Part model, mm, in its own coordinate system. Face numbers are marked on the shaded views. A direction names the side the tool comes from. Round coordinates to 2 decimals unless told otherwise and drop trailing zeros. Order: outer loops, then holes, each group sorted by start corner. A loop starts at its lowest first (then second) coordinate and runs counter-clockwise, first axis right, second up. Notation, with made-up numbers: (40.5, 67.5) -> (48.5, 67.5) arc R23 ccw to (48.5, 75.5) -> close; hole circle Ø9 at (88, -15.5). An arc over 180 degrees is marked (long way). Use CSV: the item, a comma, the result in double quotes.
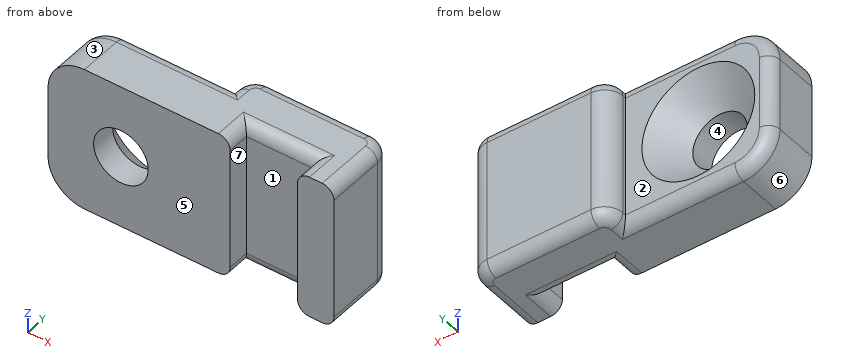
```python
from build123d import *

# Parameters (mm, degrees)
RESSALTO_EXTRUS_O1_DEPTH = 8
ESBO_O2_R                = 1.5
CORTE_EXTRUS_O1_DEPTH    = 6
CHANFRO2_SIZE            = 1.6
FILETE3_R                = 2
FILETE5_R                = 1
FILETE6_R                = 0.65


with BuildPart() as part:
    # Esboço1 → Ressalto-extrusão1 (new body)
    with BuildSketch(Plane.XY):
        Polygon((-11.5, -1.2), (-11.5, 1.8), (-3.5, 1.8), (-3.5, 3), (4.2, 3), (4.2, -1.2), (2.2, -1.2), (2.2, 0), (-1.5, 0), (-1.5, -1.2), align=None)
    extrude(amount=RESSALTO_EXTRUS_O1_DEPTH)

    # Esboço2 → Corte-extrusão1 (cut)
    with BuildSketch(Plane(origin=(0, 1.8, 0), x_dir=(1, 0, 0), z_dir=(0, 1, 0))):
        with Locations(Location((-7.5, -4, 0), (0, 0, 180))):
            Circle(ESBO_O2_R)
    extrude(amount=-CORTE_EXTRUS_O1_DEPTH, mode=Mode.SUBTRACT)

    # Chanfro2
    chanfro2_edges = [part.edges().sort_by_distance(p)[0] for p in [
        (-6, 1.8, 4),
    ]]
    chamfer(chanfro2_edges, length=CHANFRO2_SIZE)

    # Filete3
    filete3_edges = [part.edges().sort_by_distance(p)[0] for p in [
        (-11.5, 0.3, 0),
        (-11.5, 0.3, 8),
    ]]
    fillet(filete3_edges, radius=FILETE3_R)

    # Filete5
    filete5_edges = [part.edges().sort_by_distance(p)[0] for p in [
        (-3.5, 3, 4),
        (4.2, 3, 4),
    ]]
    fillet(filete5_edges, radius=FILETE5_R)

    # Filete6
    filete6_edges = [part.edges().sort_by_distance(p)[0] for p in [
        (-1.5, -0.6, 0),
        (-6.5, 1.8, 0),
        (4.2, 0.4, 0),
        (2.2, -0.6, 0),
        (0.35, 0, 0),
        (4.2, 0.4, 8),
        (-6.5, 1.8, 8),
        (-1.5, -0.6, 8),
        (-11.5, 1.8, 4),
        (-10.914213562, 1.8, 0.585786438),
        (-10.914213562, 1.8, 7.414213562),
        (0.35, 0, 8),
        (-3.5, 1.9, 0),
        (-3.5, 1.9, 8),
        (0.35, 3, 0),
        (3.907106781, 2.707106781, 0),
        (-3.207106781, 2.707106781, 0),
        (0.35, 3, 8),
        (3.907106781, 2.707106781, 8),
        (-3.207106781, 2.707106781, 8),
        (2.2, -0.6, 8),
    ]]
    fillet(filete6_edges, radius=FILETE6_R)


solid = part.part
```
(1) Cut at A-A, the plane y = -0.2. Give the cut face in (x, z).
Reply:
outline,"(-11.5, 2) arc R2 ccw to (-9.5, 0) -> (-2.15, 0) arc R0.65 ccw to (-1.5, 0.65) -> (-1.5, 7.35) arc R0.65 ccw to (-2.15, 8) -> (-9.5, 8) arc R2 ccw to (-11.5, 6) -> close; (2.2, 0.65) arc R0.65 ccw to (2.85, 0) -> (3.55, 0) arc R0.65 ccw to (4.2, 0.65) -> (4.2, 7.35) arc R0.65 ccw to (3.55, 8) -> (2.85, 8) arc R0.65 ccw to (2.2, 7.35) -> close; hole circle Ø3 at (-7.5, 4)"
(2) Cut at D-D, the plane x = 1.5. Give the cut face in (y, z).
Reply:
outline,"(0, 0.65) arc R0.65 ccw to (0.65, 0) -> (2.35, 0) arc R0.65 ccw to (3, 0.65) -> (3, 7.35) arc R0.65 ccw to (2.35, 8) -> (0.65, 8) arc R0.65 ccw to (0, 7.35) -> close"
(3) Cut at C-C, the plane z = 4. Give the cut face in (x, y).
Reply:
outline,"(-11.5, -1.2) -> (-9, -1.2) -> (-9, 0.2) -> (-10.6, 1.8) -> (-10.85, 1.8) arc R0.65 ccw to (-11.5, 1.15) -> close; (-6, -1.2) -> (-1.5, -1.2) -> (-1.5, 0) -> (2.2, 0) -> (2.2, -1.2) -> (4.2, -1.2) -> (4.2, 2) arc R1 ccw to (3.2, 3) -> (-2.5, 3) arc R1 ccw to (-3.5, 2) -> (-3.5, 1.8) -> (-4.4, 1.8) -> (-6, 0.2) -> close"
(4) Cut at B-B, the plane x = -7.5. Give the cut face in (y, z), then the cut area to 3 significant figures.
Reply:
outline,"(-1.2, 0) -> (1.15, 0) arc R0.65 ccw to (1.8, 0.65) -> (1.8, 0.9) -> (0.2, 2.5) -> (-1.2, 2.5) -> close; (-1.2, 5.5) -> (0.2, 5.5) -> (1.8, 7.1) -> (1.8, 7.35) arc R0.65 ccw to (1.15, 8) -> (-1.2, 8) -> close"
area,"12.3 mm2"
(5) Pull direction X, two halves, no side cores. Call the marked faces 4, 5, 6 and 7: released by +X, released by -X, zero draft, split by the parting line, or undercut.
Reply:
face 4,"undercut"
face 5,"zero draft"
face 6,"released by -X"
face 7,"undercut"
(6) Which spindle directions (+Z, -Z, +X, -X, +Y, -Y) get a long thin tool onto all of the face, cutting with end or side? Do the marked faces 1, 2 and 3. Say none if no direction does.
Reply:
face 1,"+Z, -Z, -Y"
face 2,"+Z, -Z, -X, +Y"
face 3,"+Z, -X, +Y, -Y"
(7) Probe probe 1 along Z at (x, y) = (-7.5, -0.3); probe 2 along X at (y, z) = (-0.5, 4.5); probe 3 along X at (y, z) = (2.05, 2). List the from-to ranges inside material, lowest first. Write a range as [from, to].
Reply:
probe 1,"[0, 2.5], [5.5, 8]"
probe 2,"[-11.5, -8.91], [-6.09, -1.5], [2.2, 4.2]"
probe 3,"[-3.5, 4.2]"
(8) Drop a flat-ended pin along its axis: P1, Ø4, axis at x = -8.5, z = 3, coming from the -Y side. Give the stop position or say it passes through.
Reply:
P1,"y = -1.2"
